```python
from build123d import *

# Parameters (mm, degrees)
BOX_W             = 20
BOX_H             = 25.5
BOX_DEPTH         = 28.42
BOX001_W          = 2
BOX001_H          = 7
BOX001_DEPTH      = 31.5
BOX002_W          = 2
BOX002_H          = 7.5
BOX002_DEPTH      = 31
BOX003_W          = 21
BOX003_H          = 19
BOX003_DEPTH      = 6
BOX008_W          = 18
BOX008_H          = 7
BOX008_DEPTH      = 9.5
BOX009_W          = 22
BOX009_H          = 7
BOX009_DEPTH      = 3.175
BOX010_W          = 23
BOX010_H          = 7
BOX010_DEPTH      = 3.2
BOX011_W          = 1
BOX011_H          = 1
BOX011_DEPTH      = 24
BOX012_W          = 1
BOX012_H          = 1
BOX012_DEPTH      = 24
BOX019_W          = 21
BOX019_H          = 20
BOX019_DEPTH      = 3
BOX020_W          = 1
BOX020_H          = 1
BOX020_DEPTH      = 8.2
BOX021_W          = 1
BOX021_H          = 1
BOX021_DEPTH      = 24
BOX022_W          = 1
BOX022_H          = 1
BOX022_DEPTH      = 24
CYLINDER_R        = 0.5
CYLINDER_DEPTH    = 19
CYLINDER001_R     = 0.5
CYLINDER001_DEPTH = 24
CYLINDER002_R     = 0.5
CYLINDER002_DEPTH = 17
CYLINDER003_R     = 0.5
CYLINDER003_DEPTH = 17
BOX023_W          = 1
BOX023_H          = 1
BOX023_DEPTH      = 24
BOX024_W          = 1
BOX024_H          = 1
BOX024_DEPTH      = 24
BOX025_W          = 1
BOX025_H          = 1
BOX025_DEPTH      = 24
BOX026_W          = 1
BOX026_H          = 1
BOX026_DEPTH      = 24
BOX027_W          = 1
BOX027_H          = 1
BOX027_DEPTH      = 24
BOX028_W          = 1
BOX028_H          = 1
BOX028_DEPTH      = 24
BOX029_W          = 2
BOX029_H          = 8
BOX029_DEPTH      = 8
BOX030_W          = 2
BOX030_H          = 8
BOX030_DEPTH      = 8
BOX033_W          = 2
BOX033_H          = 7
BOX033_DEPTH      = 2
BOX034_W          = 2
BOX034_H          = 7
BOX034_DEPTH      = 2
CYLINDER006_R     = 1
CYLINDER006_DEPTH = 7
BOX035_W          = 0.8
BOX035_H          = 7
BOX035_DEPTH      = 2
BOX036_W          = 1
BOX036_H          = 1
BOX036_DEPTH      = 7
CYLINDER007_R     = 1
CYLINDER007_DEPTH = 7
BOX037_W          = 0.8
BOX037_H          = 7
BOX037_DEPTH      = 2
BOX038_W          = 1
BOX038_H          = 1
BOX038_DEPTH      = 7
FILLET008_R       = 3


with BuildPart() as part:
    # Box → Box (join)
    with BuildSketch(Plane(origin=(-10, 0, 0), x_dir=(1, 0, 0), z_dir=(0, 0, 1))):
        with Locations((10, 12.75)):
            Rectangle(BOX_W, BOX_H)
    extrude(amount=BOX_DEPTH)

    # Box001 → Box001 (cut)
    with BuildSketch(Plane(origin=(-10, 18.5, 0), x_dir=(1, 0, 0), z_dir=(0, 0, 1))):
        with Locations((1, 3.5)):
            Rectangle(BOX001_W, BOX001_H)
    extrude(amount=BOX001_DEPTH, mode=Mode.SUBTRACT)

    # Box002 → Box002 (cut)
    with BuildSketch(Plane(origin=(8, 18.5, 0), x_dir=(1, 0, 0), z_dir=(0, 0, 1))):
        with Locations((1, 3.75)):
            Rectangle(BOX002_W, BOX002_H)
    extrude(amount=BOX002_DEPTH, mode=Mode.SUBTRACT)

    # Box003 → Box003 (cut)
    with BuildSketch(Plane(origin=(-10.5, 6.5, 10.7), x_dir=(1, 0, 0), z_dir=(0, 0, 1))):
        with Locations((10.5, 9.5)):
            Rectangle(BOX003_W, BOX003_H)
    extrude(amount=BOX003_DEPTH, mode=Mode.SUBTRACT)

    # Box008 → Box008 (cut)
    with BuildSketch(Plane(origin=(-9, 18.5, 9.45), x_dir=(1, 0, 0), z_dir=(0, 0, 1))):
        with Locations((9, 3.5)):
            Rectangle(BOX008_W, BOX008_H)
    extrude(amount=BOX008_DEPTH, mode=Mode.SUBTRACT)

    # Box009 → Box009 (cut)
    with BuildSketch(Plane(origin=(-11, 18.5, 0), x_dir=(1, 0, 0), z_dir=(0, 0, 1))):
        with Locations((11, 3.5)):
            Rectangle(BOX009_W, BOX009_H)
    extrude(amount=BOX009_DEPTH, mode=Mode.SUBTRACT)

    # Box010 → Box010 (cut)
    with BuildSketch(Plane(origin=(-11.5, 18.5, 25.3), x_dir=(1, 0, 0), z_dir=(0, 0, 1))):
        with Locations((11.5, 3.5)):
            Rectangle(BOX010_W, BOX010_H)
    extrude(amount=BOX010_DEPTH, mode=Mode.SUBTRACT)

    # Box011 → Box011 (cut)
    with BuildSketch(Plane(origin=(-0.5, 1.95, 0), x_dir=(1, 0, 0), z_dir=(0, 0, 1))):
        with Locations((0.5, 0.5)):
            Rectangle(BOX011_W, BOX011_H)
    extrude(amount=BOX011_DEPTH, mode=Mode.SUBTRACT)

    # Box012 → Box012 (cut)
    with BuildSketch(Plane(origin=(2.27, 2.1, 0), x_dir=(1, 0, 0), z_dir=(0, 0, 1))):
        with Locations((0.5, 0.5)):
            Rectangle(BOX012_W, BOX012_H)
    extrude(amount=BOX012_DEPTH, mode=Mode.SUBTRACT)

    # Box019 → Box019 (cut)
    with BuildSketch(Plane(origin=(-10.5, 0, 26.55), x_dir=(1, 0, 0), z_dir=(0, 0, 1))):
        with Locations((10.5, 10)):
            Rectangle(BOX019_W, BOX019_H)
    extrude(amount=BOX019_DEPTH, mode=Mode.SUBTRACT)

    # Box020 → Box020 (cut)
    with BuildSketch(Plane(origin=(-0.5, 8.4, 0), x_dir=(1, 0, 0), z_dir=(0, 0, 1))):
        with Locations((0.5, 0.5)):
            Rectangle(BOX020_W, BOX020_H)
    extrude(amount=BOX020_DEPTH, mode=Mode.SUBTRACT)

    # Box021 → Box021 (cut)
    with BuildSketch(Plane(origin=(4.975, 2.1, 0), x_dir=(1, 0, 0), z_dir=(0, 0, 1))):
        with Locations((0.5, 0.5)):
            Rectangle(BOX021_W, BOX021_H)
    extrude(amount=BOX021_DEPTH, mode=Mode.SUBTRACT)

    # Box022 → Box022 (cut)
    with BuildSketch(Plane(origin=(-5.975, 2.1, 0), x_dir=(1, 0, 0), z_dir=(0, 0, 1))):
        with Locations((0.5, 0.5)):
            Rectangle(BOX022_W, BOX022_H)
    extrude(amount=BOX022_DEPTH, mode=Mode.SUBTRACT)

    # Cylinder → Cylinder (cut)
    with BuildSketch(Plane(origin=(0, 28, 7.7), x_dir=(1, 0, 0), z_dir=(0, -1, 0))):
        Circle(CYLINDER_R)
    extrude(amount=CYLINDER_DEPTH, mode=Mode.SUBTRACT)

    # Cylinder001 → Cylinder001 (cut)
    with BuildSketch(Plane(origin=(0, 2, 23.55), x_dir=(1, 0, 0), z_dir=(0, 1, 0))):
        Circle(CYLINDER001_R)
    extrude(amount=CYLINDER001_DEPTH, mode=Mode.SUBTRACT)

    # Cylinder002 → Cylinder002 (cut)
    with BuildSketch(Plane(origin=(5.475, 9.2, 7.7), x_dir=(1, 0, 0), z_dir=(0, 1, 0))):
        Circle(CYLINDER002_R)
    extrude(amount=CYLINDER002_DEPTH, mode=Mode.SUBTRACT)

    # Cylinder003 → Cylinder003 (cut)
    with BuildSketch(Plane(origin=(-5.475, 9, 7.7), x_dir=(1, 0, 0), z_dir=(0, 1, 0))):
        Circle(CYLINDER003_R)
    extrude(amount=CYLINDER003_DEPTH, mode=Mode.SUBTRACT)

    # Box023 → Box023 (cut)
    with BuildSketch(Plane(origin=(-3.275, 2.1, 0), x_dir=(1, 0, 0), z_dir=(0, 0, 1))):
        with Locations((0.5, 0.5)):
            Rectangle(BOX023_W, BOX023_H)
    extrude(amount=BOX023_DEPTH, mode=Mode.SUBTRACT)

    # Box024 → Box024 (cut)
    with BuildSketch(Plane(origin=(-3.275, 8.55, 0), x_dir=(1, 0, 0), z_dir=(0, 0, 1))):
        with Locations((0.5, 0.5)):
            Rectangle(BOX024_W, BOX024_H)
    extrude(amount=BOX024_DEPTH, mode=Mode.SUBTRACT)

    # Box025 → Box025 (cut)
    with BuildSketch(Plane(origin=(0.9, 4.65, 0), x_dir=(1, 0, 0), z_dir=(0, 0, 1))):
        with Locations((0.5, 0.5)):
            Rectangle(BOX025_W, BOX025_H)
    extrude(amount=BOX025_DEPTH, mode=Mode.SUBTRACT)

    # Box026 → Box026 (cut)
    with BuildSketch(Plane(origin=(-1.877, 4.65, 0), x_dir=(1, 0, 0), z_dir=(0, 0, 1))):
        with Locations((0.5, 0.5)):
            Rectangle(BOX026_W, BOX026_H)
    extrude(amount=BOX026_DEPTH, mode=Mode.SUBTRACT)

    # Box027 → Box027 (cut)
    with BuildSketch(Plane(origin=(3.65, 4.65, 0), x_dir=(1, 0, 0), z_dir=(0, 0, 1))):
        with Locations((0.5, 0.5)):
            Rectangle(BOX027_W, BOX027_H)
    extrude(amount=BOX027_DEPTH, mode=Mode.SUBTRACT)

    # Box028 → Box028 (cut)
    with BuildSketch(Plane(origin=(-4.6, 4.65, 0), x_dir=(1, 0, 0), z_dir=(0, 0, 1))):
        with Locations((0.5, 0.5)):
            Rectangle(BOX028_W, BOX028_H)
    extrude(amount=BOX028_DEPTH, mode=Mode.SUBTRACT)

    # Box029 → Box029 (cut)
    with BuildSketch(Plane(origin=(6.735, 18.5, 2.3), x_dir=(0.984808, 0, -0.173648), z_dir=(0.173648, 0, 0.984808))):
        with Locations((1, 4)):
            Rectangle(BOX029_W, BOX029_H)
    extrude(amount=BOX029_DEPTH, mode=Mode.SUBTRACT)

    # Box030 → Box030 (cut)
    with BuildSketch(Plane(origin=(-8.765, 18.5, 2.3), x_dir=(0.984808, 0, 0.173648), z_dir=(-0.173648, 0, 0.984808))):
        with Locations((1, 4)):
            Rectangle(BOX030_W, BOX030_H)
    extrude(amount=BOX030_DEPTH, mode=Mode.SUBTRACT)

    # Box033 → Box033 (cut)
    with BuildSketch(Plane(origin=(-8, 18.5, 7.45), x_dir=(1, 0, 0), z_dir=(0, 0, 1))):
        with Locations((1, 3.5)):
            Rectangle(BOX033_W, BOX033_H)
    extrude(amount=BOX033_DEPTH, mode=Mode.SUBTRACT)

    # Box034 → Box034 (cut)
    with BuildSketch(Plane(origin=(6, 18.5, 7.45), x_dir=(1, 0, 0), z_dir=(0, 0, 1))):
        with Locations((1, 3.5)):
            Rectangle(BOX034_W, BOX034_H)
    extrude(amount=BOX034_DEPTH, mode=Mode.SUBTRACT)

    # Cylinder006 → Cylinder006 (join)
    with BuildSketch(Plane(origin=(6.815, 25.5, 8.45), x_dir=(1, 0, 0), z_dir=(0, -1, 0))):
        Circle(CYLINDER006_R)
    extrude(amount=CYLINDER006_DEPTH)

    # Box035 → Box035 (join)
    with BuildSketch(Plane(origin=(6, 18.5, 7.45), x_dir=(1, 0, 0), z_dir=(0, 0, 1))):
        with Locations((0.4, 3.5)):
            Rectangle(BOX035_W, BOX035_H)
    extrude(amount=BOX035_DEPTH)

    # Box036 → Box036 (join)
    with BuildSketch(Plane(origin=(7.6075, 25.5, 7.25), x_dir=(0.173648, 0, 0.984808), z_dir=(0, -1, 0))):
        with Locations((0.5, 0.5)):
            Rectangle(BOX036_W, BOX036_H)
    extrude(amount=BOX036_DEPTH)

    # Cylinder007 → Cylinder007 (join)
    with BuildSketch(Plane(origin=(-6.815, 25.5, 8.45), x_dir=(1, 0, 0), z_dir=(0, -1, 0))):
        Circle(CYLINDER007_R)
    extrude(amount=CYLINDER007_DEPTH)

    # Box037 → Box037 (join)
    with BuildSketch(Plane(origin=(-6.8, 18.5, 7.45), x_dir=(1, 0, 0), z_dir=(0, 0, 1))):
        with Locations((0.4, 3.5)):
            Rectangle(BOX037_W, BOX037_H)
    extrude(amount=BOX037_DEPTH)

    # Box038 → Box038 (join)
    with BuildSketch(Plane(origin=(-7.7834, 25.5, 8.25), x_dir=(0.173648, 0, -0.984808), z_dir=(0, -1, 0))):
        with Locations((0.5, 0.5)):
            Rectangle(BOX038_W, BOX038_H)
    extrude(amount=BOX038_DEPTH)

    # Fillet008
    fillet008_edges = [part.edges().sort_by_distance(p)[0] for p in [
        (10, 9.25, 26.55),
        (-10, 9.25, 26.55),
    ]]
    fillet(fillet008_edges, radius=FILLET008_R)


solid = part.part
```
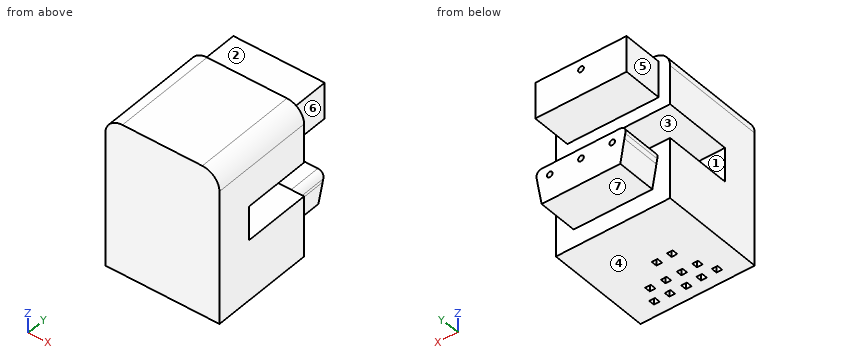
Model file for the job. Use its own axes, mm. Face numbers are marked on the shaded views. A direction names the side the tool comes from. Give positions to 0.01 mm unless a question says otherwise; leave off trailing zeros. Loops run counter-clockwise (first coordinate to the right, second up) from the corner with the lowest first, then second, coordinate; pieces in that order, holes last. Notation, with made-up numbers: (58, 62.5) - (85, 62.5) arc R24 ccw to (85, 80.5) - close; hole circle Ø2 at (9, 7.25). An arc over 180 degrees is marked (long way). One line per item, written item: value. Start each with the question number.
1. Slice it at A-A (y = 15.5). List the corners of the cut face in (x, z) (3 decimals), plus the area to 3 significant figures.
2. Slice it at B-B (x = -4). List the corners of the cut face in (y, z) (3 decimals), plus the area to 3 significant figures.
3. Which spindle directions (+Z, -Z, +X, -X, +Y, -Y) get a long thin tool onto all of the face, cutting with end or side? Do the marked faces 5, 6 and 7. Say none if no direction does.
4. Probe L1, parallel to X at y = 13.25, z = 7.7 (3 decimals); L2, parallel to Z at x = 0, y = 16.5; L3, parallel to Z at x = 0, y = 18.75 (3 decimals). List the from-to ranges inside material, lowest first. Write a range as from..to.
5. Slice it at C-C (z = 19.5). Give the number of separate pieces and of enclosed holes in the cut face, plus the area to 3 significant figures.
6. Pin check, flat tips, straight feed: pin 1 (0.8 mm diameter, centred on x = 0, z = 2, fed in from -Y); pin 2 (3 mm diameter, centred on y = 15.5, z = 14, fed in from -X); pin 3 (7.5 mm diameter, centred on x = 2, y = 23.5, fed in from -Z) (3 decimals); pin 4 (0.8 mm diameter, centred on x = 0, y = 2.5, fed in from -Z). Stop position of each tip, or through.
7. Pull direction Z, two halves, no side cores. Call the marked faces 1, 2, 3 and 4: pulls with the +Z half, pulls with the -Z half, needs draft (parallel to the pull), parting line crosses it, or undercut.
8. Slice it at D-D (y = 2.5). List the corners of the cut face in (x, z) (3 decimals), plus the area to 3 significant figures.
Solution:
1. outline: (-10, 0) - (10, 0) - (10, 10.7) - (-10, 10.7) - close; (-10, 16.7) - (10, 16.7) - (10, 23.55) arc R3 ccw to (7, 26.55) - (-7, 26.55) arc R3 ccw to (-10, 23.55) - close; hole circle Ø1 at (-5.475, 7.7); hole circle Ø1 at (0, 7.7); hole circle Ø1 at (0, 23.55); hole circle Ø1 at (5.475, 7.7)
1. area: 404 mm^2
2. outline: (0, 0) - (4.65, 0) - (4.65, 24) - (5.65, 24) - (5.65, 0) - (18.5, 0) - (18.5, 3.175) - (25.5, 3.175) - (25.5, 9.45) - (18.5, 9.45) - (18.5, 10.7) - (6.5, 10.7) - (6.5, 16.7) - (18.5, 16.7) - (18.5, 18.95) - (25.5, 18.95) - (25.5, 25.3) - (18.5, 25.3) - (18.5, 26.55) - (0, 26.55) - close
2. area: 484 mm^2
3. face 5: +Z, -Z, -X, +Y
3. face 6: +Z, -Z, +X, +Y
3. face 7: -Z, +X, -X, +Y
4. L1: x = -10..-5.975, -4.975..-0.5, 0.5..4.975, 5.975..10
4. L2: z = 0..7.2, 8.2..10.7, 16.7..23.05, 24.05..26.55
4. L3: z = 3.175..7.2, 8.2..9.45, 18.95..23.05, 24.05..25.3
5. separate pieces: 1
5. enclosed holes: 10
5. area: 472 mm^2
6. pin 1: stops at y = 0
6. pin 2: passes through
6. pin 3: stops at z = 3.175
6. pin 4: stops at z = 24
7. face 1: undercut
7. face 2: pulls with the +Z half
7. face 3: undercut
7. face 4: pulls with the -Z half
8. outline: (-10, 0) - (-5.975, 0) - (-5.975, 24) - (-4.975, 24) - (-4.975, 0) - (-3.275, 0) - (-3.275, 24) - (-2.275, 24) - (-2.275, 0) - (-0.5, 0) - (-0.5, 24) - (-0.218, 24) arc R0.5 cw to (0.218, 24) - (0.5, 24) - (0.5, 0) - (2.27, 0) - (2.27, 24) - (3.27, 24) - (3.27, 0) - (4.975, 0) - (4.975, 24) - (5.975, 24) - (5.975, 0) - (10, 0) - (10, 23.55) arc R3 ccw to (7, 26.55) - (-7, 26.55) arc R3 ccw to (-10, 23.55) - close
8. area: 407 mm^2
